The drawing under review shows one solid part. Ordinate dimensions are in mm from its lowest x, y, z. Coordinates: 2 decimals unless noted, no trailing zeros. Loops run counter-clockwise (first coordinate to the right, second up) from the corner with the lowest first, then second, coordinate; pieces in that order, holes last. Notation, with made-up numbers: (58.25, -15.75) -> (109.25, -15.75) arc R30 cw to (109.25, 20.25) -> close; hole circle Ø10 at (52.5, 3.5). An arc over 180 degrees is marked (long way). Use a Markdown table: item, result.
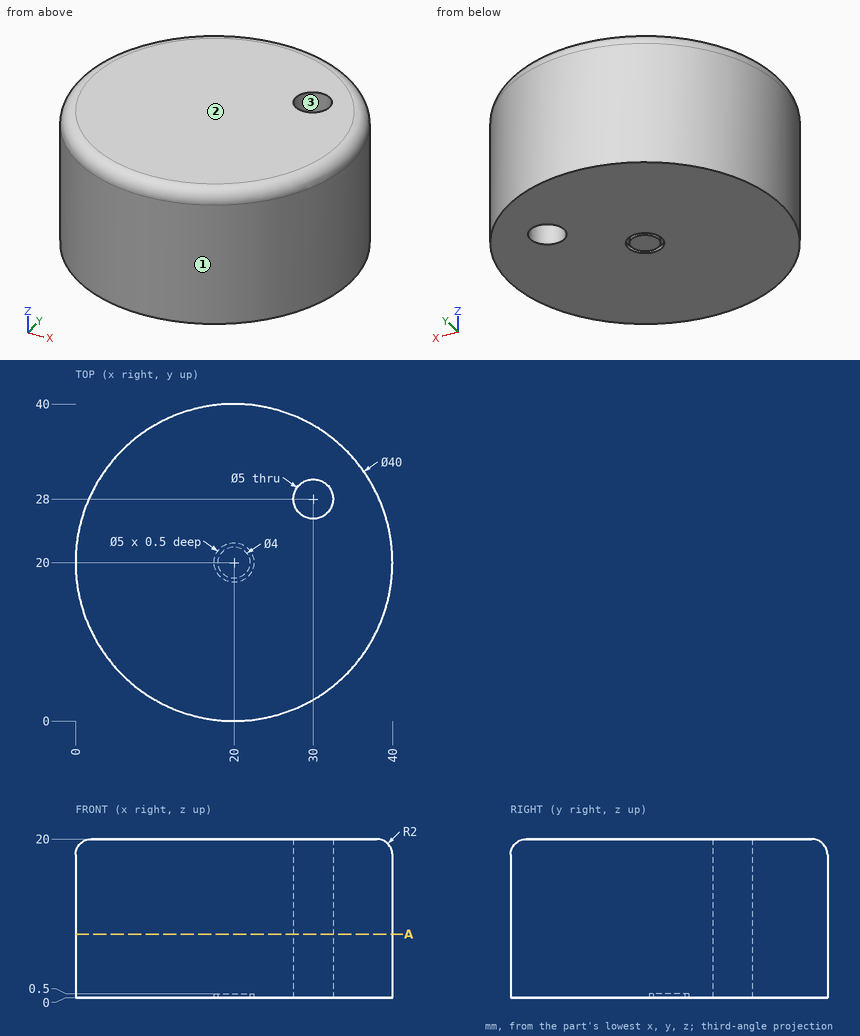
(1) Mouldability with a two-part tool opening along Y and no side actions: class the marked faces 1, 2 and 3 as pulls with the +Y half, pulls with the -Y half, needs draft (parallel to the pull), parting line crosses it, or undercut.
Found:
| item | result |
|---|---|
| face 1 | parting line crosses it |
| face 2 | needs draft |
| face 3 | undercut |
(2) For pin 1 Ø8 at (x, z) = (18.5, 5.5) entering from -Y; pin 2 Ø4 at (x, y) = (21, 19.5) entering from -Z; pin 3 Ø8 at (y, z) = (27, 3) entering from +X; pin 4 Ø3 at (x, z) = (24, 3.5) entering from -Y, all flat-tipped, find the tip position at first contact; note any pin that passes through.
Found:
| item | result |
|---|---|
| pin 1 | stops at y = 0 |
| pin 2 | stops at z = 0 |
| pin 3 | stops at x = 39.77 |
| pin 4 | stops at y = 0.16 |
(3) For line 1 along Y through (x, z) = (20, 0.15); line 2 along X through (y, z) = (28, 13.75); line 3 along X through (y, z) = (29, 3.75), list the stretches that pass through material, from the lowest coordinate up.
Found:
| item | result |
|---|---|
| line 1 | y = 0 to 17.5, 18 to 22, 22.5 to 40 |
| line 2 | x = 1.67 to 27.5, 32.5 to 38.33 |
| line 3 | x = 2.14 to 27.71, 32.29 to 37.86 |
(4) Take a section at A-A on z = 8. Write out the cut boundary in (x, y).
Found:
| item | result |
|---|---|
| outline | circle Ø40 at (20, 20); hole circle Ø5 at (30, 28) |
